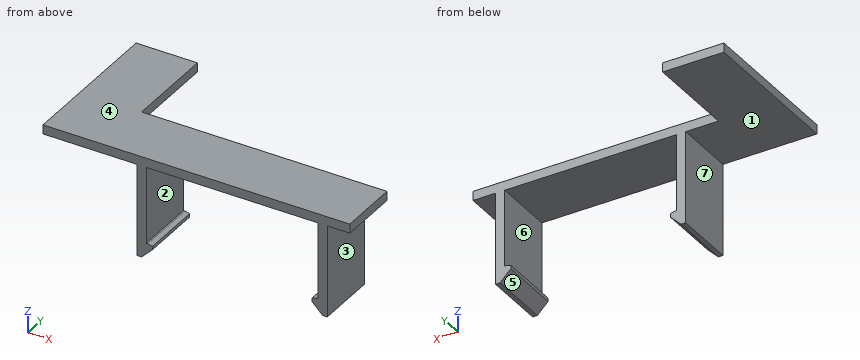
```python
from build123d import *

# Parameters (mm, degrees)
BOSS_EXTRU_1_DEPTH            = 3
ESQUISSE2_W                   = 3
ESQUISSE2_H                   = 20
BOSS_EXTRU_2_DEPTH            = 30
ESQUISSE3_W                   = 5
ESQUISSE3_H                   = 20
BOSS_EXTRU_3_DEPTH            = 2
CHANFREIN1_SIZE               = 3.5
CHANFREIN2_SIZE               = 1.5
CHANFREIN2_SIZE2              = 0.401923789
CHANFREIN1_OF_SYM_TRIE1_SIZE  = 3.5
CHANFREIN2_OF_SYM_TRIE1_SIZE2 = 1.5
CHANFREIN2_OF_SYM_TRIE1_SIZE  = 0.401923789


with BuildPart() as part:
    # Esquisse1 → Boss.-Extru.1 (new body)
    with BuildSketch(Plane.XY):
        Polygon((-50, 0), (-50, -50), (50, -50), (50, -30), (-30, -30), (-30, 0), align=None)
    extrude(amount=BOSS_EXTRU_1_DEPTH)

    # Esquisse2 → Boss.-Extru.2 (add)
    with BuildSketch(Plane(origin=(0, 0, 0), x_dir=(-1, 0, 0), z_dir=(0, 0, -1))):
        with Locations((-41.161947113, -40)):
            Rectangle(ESQUISSE2_W, ESQUISSE2_H)
    boss_extru_2 = extrude(amount=BOSS_EXTRU_2_DEPTH)

    # Esquisse3 → Boss.-Extru.3 (add)
    with BuildSketch(Plane.ZY.offset(-39.661947113)):
        with Locations((-27.5, -40)):
            Rectangle(ESQUISSE3_W, ESQUISSE3_H)
    boss_extru_3 = extrude(amount=BOSS_EXTRU_3_DEPTH)

    # Chanfrein1
    chanfrein1_edges = [part.edges().sort_by_distance(p)[0] for p in [
        (37.661947113, -40, -30),
    ]]
    chamfer(chanfrein1_edges, length=CHANFREIN1_SIZE)

    # Chanfrein2
    chanfrein2_edges = [part.edges().sort_by_distance(p)[0] for p in [
        (37.661947113, -40, -25),
    ]]
    chanfrein2_side = [part.faces().sort_by_distance(p)[0] for p in [
        (38.661947113, -40, -25),
    ]]
    chamfer(chanfrein2_edges, length=CHANFREIN2_SIZE, length2=CHANFREIN2_SIZE2, reference=chanfrein2_side[0])

    # Symétrie1: Boss.-Extru.2, Boss.-Extru.3 across plane
    add(boss_extru_2.mirror(Plane.ZY.offset(-11.661947113)))
    add(boss_extru_3.mirror(Plane.ZY.offset(-11.661947113)))

    # Chanfrein1 of Symétrie1
    chanfrein1_of_sym_trie1_edges = [part.edges().sort_by_distance(p)[0] for p in [
        (-14.338052887, -40, -30),
    ]]
    chamfer(chanfrein1_of_sym_trie1_edges, length=CHANFREIN1_OF_SYM_TRIE1_SIZE)

    # Chanfrein2 of Symétrie1
    chanfrein2_of_sym_trie1_edges = [part.edges().sort_by_distance(p)[0] for p in [
        (-14.338052887, -40, -25),
    ]]
    chamfer(chanfrein2_of_sym_trie1_edges, length=CHANFREIN2_OF_SYM_TRIE1_SIZE, length2=CHANFREIN2_OF_SYM_TRIE1_SIZE2)


solid = part.part
```
Could you check a few things on this model? Use its own coordinates, in mm. Face numbers are marked on the shaded views. A direction names the side the tool comes from. Round coordinates to 2 decimals unless told otherwise and drop trailing zeros. Loops run counter-clockwise (first coordinate to the right, second up) from the corner with the lowest first, then second, coordinate; pieces in that order, holes last.
Q1. Thinking about a two-plate mould opening in X: for the marked faces 1, 2 and 3, which applies, pulls with the +X half, pulls with the -X half, needs draft (parallel to the pull), parting line crosses it, or undercut?
Q2. I want a section at C-C (x = 25.5). Write out the boundary of the cut face in (y, z).
Q3. I want a section at A-A (z = -12). Write out the boundary of the cut face in (x, y), and give its area (3 significant figures).
Q4. On a 3-axis mill with a long thin cutter (end or side, diameter ignored), from which of +Z, -Z, +X, -X, +Y, -Y can I reach the whole of each face in a straight line? I mean the marked faces 4, 5, 6 and 7. Say none if no direction works.
Q5. Please list where these lines run through material, in increasing order: L1, parallel to X at y = -39, z = -6; L2, parallel to Z at x = -10.5, y = -35.
Q6. For P1, Ø1.2, axis at y = -43, z = -26, coming from the -X side; P2, Ø1, axis at y = -41, z = -2, coming from the +X side; P3, Ø15.5, axis at x = -40.5, y = -27, coming from the -Z side; P4, Ø6, axis at x = 45.5, y = -36.5, coming from the -Z side, each with a flat end and sliding along its axis, tell me the tip position at first contact or that it passes through.
Q7. I want a section at B-B (y = -35). Write out the boundary of the cut face in (x, z).
Answer below:
1. face 1: needs draft
1. face 2: undercut
1. face 3: pulls with the +X half
2. outline: (-50, 0) - (-30, 0) - (-30, 3) - (-50, 3) - close
3. outline: (-19.34, -50) - (-16.34, -50) - (-16.34, -30) - (-19.34, -30) - close; (39.66, -50) - (42.66, -50) - (42.66, -30) - (39.66, -30) - close
3. area: 120 mm2
4. face 4: +Z, +X, -X, +Y, -Y
4. face 5: -Z, +Y, -Y
4. face 6: +Y, -Y
4. face 7: -Z, -X, +Y, -Y
5. L1: x = -19.34 to -16.34, 39.66 to 42.66
5. L2: z = 0 to 3
6. P1: stops at x = -19.34
6. P2: stops at x = 42.66
6. P3: stops at z = 0
6. P4: stops at z = -30
7. outline: (-50, 0) - (-19.34, 0) - (-19.34, -30) - (-17.84, -30) - (-14.34, -26.5) - (-14.34, -25.4) - (-15.84, -25) - (-16.34, -25) - (-16.34, 0) - (39.66, 0) - (39.66, -25) - (39.16, -25) - (37.66, -25.4) - (37.66, -26.5) - (41.16, -30) - (42.66, -30) - (42.66, 0) - (50, 0) - (50, 3) - (-50, 3) - close
